Could you check a few things on this model? Use its own coordinates, in mm. Round coordinates to 2 decimals unless told otherwise and drop trailing zeros. Write each loop counter-clockwise with the first axis right and the second up, starting at its lowest first coordinate (ties: lowest second). Pieces come first, ordered by that corner, then holes.
```python
from build123d import *

# Parameters (mm, degrees)
SKETCH1_W           = 50
SKETCH1_H           = 6
BOSS_EXTRUDE1_DEPTH = 4
SKETCH2_R           = 1.45
CUT_EXTRUDE1_DEPTH  = 51.517323761
FILLET1_R           = 2.5
SKETCH3_R           = 1.45
CUT_EXTRUDE2_DEPTH  = 51.517323761


with BuildPart() as part:
    # Sketch1 → Boss-Extrude1 (new body)
    with BuildSketch(Plane.XY):
        with Locations((-25, -3)):
            Rectangle(SKETCH1_W, SKETCH1_H)
    extrude(amount=BOSS_EXTRUDE1_DEPTH)

    # Sketch2 → Cut-Extrude1 (cut, through all)
    with BuildSketch(Plane(origin=(0, 0, 0), x_dir=(-1, 0, 0), z_dir=(0, 0, -1))):
        with Locations((3, -3)):
            Circle(SKETCH2_R)
        with Locations((37, -3)):
            Circle(SKETCH2_R)
    extrude(amount=-CUT_EXTRUDE1_DEPTH, mode=Mode.SUBTRACT)

    # Fillet1
    fillet1_edges = [part.edges().sort_by_distance(p)[0] for p in [
        (0, -6, 2),
        (-50, -6, 2),
        (-50, 0, 2),
        (0, 0, 2),
    ]]
    fillet(fillet1_edges, radius=FILLET1_R)

    # Sketch3 → Cut-Extrude2 (cut, through all)
    with BuildSketch(Plane(origin=(0, 0, 0), x_dir=(-1, 0, 0), z_dir=(0, 0, -1))):
        with Locations((47, -3)):
            Circle(SKETCH3_R)
    extrude(amount=-CUT_EXTRUDE2_DEPTH, mode=Mode.SUBTRACT)


solid = part.part
```
Q1. If I drill on L1, parallel to Y at x = -47, z = 2.1; L2, parallel to X at y = -3.75, z = 3.85; L3, parallel to X at y = -2.75, z = 3.35, over which ranges is the centre line in solid material (lowest first)?
Q2. Imagine slicing it at C-C, the plane x = -37.5. Write out the boundary of the cut face in (y, z).
Q3. Imagine slicing it at D-D, the plane y = -5. Write out the boundary of the cut face in (x, z).
Q4. We'd pull the mould along Y, two halves only. Please class faces 1 (the flat face through (-25, -3, 4)), 2 (the cylindrical face through (-0.752, -5.287, 2.028)), 3 (the cylindrical face through (-35.55, -2.94, 1.97)): pulls with the +Y half, pulls with the -Y half, needs draft (parallel to the pull), parting line crosses it, or undercut.
Q5. Imagine slicing it at B-B, the plane z = 2.25. Write out the boundary of the cut face in (x, y).
Q6. Imagine slicing it at A-A, the plane x = -47. Write out the boundary of the cut face in (y, z).
Q7. I'm going to push a flat-ended pin straight in: pin 1 Ø3.5 at (x, y) = (-3, -3) entering from +Z. Where does the tip first touch, or does it pass through?
Results found:
1. L1: y = -6 to -4.45, -1.55 to 0
1. L2: x = -49.99 to -48.24, -45.76 to -38.24, -35.76 to -4.24, -1.76 to -0.01
1. L3: x = -50 to -48.43, -45.57 to -38.43, -35.57 to -4.43, -1.57 to 0
2. outline: (-6, 0) - (-4.36, 0) - (-4.36, 4) - (-6, 4) - close; (-1.64, 0) - (0, 0) - (0, 4) - (-1.64, 4) - close
3. outline: (-49.5, 0) - (-0.5, 0) - (-0.5, 4) - (-49.5, 4) - close
4. face 1: needs draft
4. face 2: pulls with the -Y half
4. face 3: undercut
5. outline: (-50, -3.5) arc R2.5 ccw to (-47.5, -6) - (-2.5, -6) arc R2.5 ccw to (0, -3.5) - (0, -2.5) arc R2.5 ccw to (-2.5, 0) - (-47.5, 0) arc R2.5 ccw to (-50, -2.5) - close; hole circle Ø2.9 at (-47, -3); hole circle Ø2.9 at (-37, -3); hole circle Ø2.9 at (-3, -3)
6. outline: (-6, 0) - (-4.45, 0) - (-4.45, 4) - (-6, 4) - close; (-1.55, 0) - (0, 0) - (0, 4) - (-1.55, 4) - close
7. pin 1: stops at z = 4
